Check sheet for the modelled part. Datum: model origin and axes. Units: mm. Face numbers are marked on the shaded views. A direction names the side the tool comes from. Round coordinates to 2 decimals unless told otherwise and drop trailing zeros. Order: outer loops, then holes, each group sorted by start corner. A loop starts at its lowest first (then second) coordinate and runs counter-clockwise, first axis right, second up. Notation, with made-up numbers: (-3.5, -11.5) -> (53.5, -11.5) arc R20 ccw to (53.5, 6.5) -> close; hole circle Ø9 at (89.25, 35.25). An arc over 180 degrees is marked (long way). Answer as CSV lines item,"result". Start each with the question number.
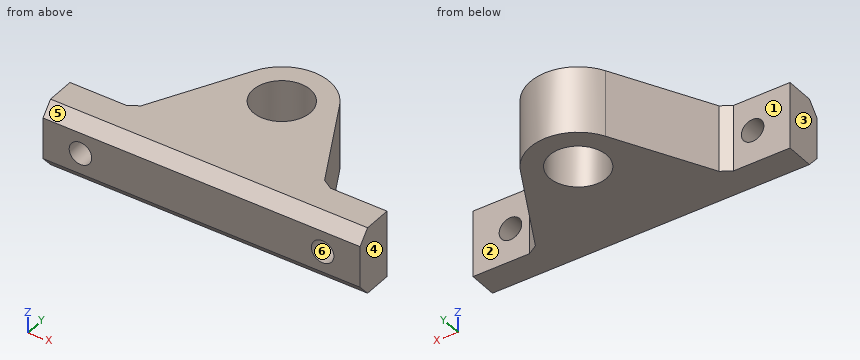
from build123d import *

# Parameters (mm, degrees)
SKETCH_R     = 4.06
PAD_DEPTH    = 9.48
PAD001_DEPTH = 45
SKETCH002_R  = 1.6
POCKET_DEPTH = 23.37485
CHAMFER_SIZE = 1


with BuildPart() as part:
    # Sketch → Pad (new body)
    with BuildSketch(Plane.XY):
        with BuildLine():
            ThreePointArc((6.02785, 14.177039), (0, 17.81385), (-6.02785, 14.177039))
            Line((-6.02785, 14.177039), (-13.5, 0))
            Line((-13.5, 0), (-22.5, 0))
            Line((-22.5, 0), (-22.5, -4))
            Line((-22.5, -4), (22.5, -4))
            Line((22.5, -4), (22.5, 0))
            Line((22.5, 0), (13.5, 0))
            Line((6.02785, 14.177039), (13.5, 0))
        make_face()
        with Locations((0, 11)):
            Circle(SKETCH_R, mode=Mode.SUBTRACT)
    extrude(amount=PAD_DEPTH)

    # Sketch001 (on Face4 of Pad) → Pad001 (join)
    with BuildSketch(Plane(origin=(-22.5, 0, 0), x_dir=(0, -1, 0), z_dir=(-1, 0, 0))):
        Polygon((4, 9.48), (4, 0), (5.56, 1.8), (5.56, 7.68), align=None)
    extrude(amount=-PAD001_DEPTH)

    # Sketch002 (on Face14 of Pad001) → Pocket (cut, through all)
    with BuildSketch(Plane.XZ.offset(5.56)):
        with Locations((-17.186, 4.74)):
            Circle(SKETCH002_R)
        with Locations((17.186, 4.74)):
            Circle(SKETCH002_R)
    extrude(amount=-POCKET_DEPTH, mode=Mode.SUBTRACT)

    # Chamfer
    chamfer_edges = [part.edges().sort_by_distance(p)[0] for p in [
        (13.5, 0, 4.74),
        (-13.5, 0, 4.74),
    ]]
    chamfer(chamfer_edges, length=CHAMFER_SIZE)


solid = part.part
1) Section check C-C on z = 7. Record the cut outline in (x, y), then the cut area to 3 significant figures.
2) Material ranges on line 1 along Y through (x, z) = (0, 2.75); line 2 along Y through (x, z) = (3, 0.5); line 3 along Y through (x, z) = (-16.5, 3), recorded low to high.
3) Section check B-B on x = 0. Record the cut outline in (y, z).
4) Section check D-D on y = -3.25. Record the cut outline in (x, z).
5) Access from +Z, -Z, +X, -X, +Y, -Y to the whole of each face (thin tool, end or side, straight path). Record for the marked faces 1, 2 and 3.
6) Section check A-A on z = 4. Record the cut outline in (x, y), then the cut area to 3 significant figures.
7) Mould release check, pull along X, two halves, no side actions. Record for the marked faces 4, 5 and 6: released by +X, released by -X, zero draft, split by the parting line, or undercut.
8) Depth check by flat-ended pin: pin 1 Ø5 at (x, z) = (-17.186, 4.74) entering from +Y; pin 2 Ø2 at (y, z) = (3.5, 1.5) entering from +X; pin 3 Ø2 at (y, z) = (12, 6.5) entering from +X. Enter the tip coordinate at first touch or a pass-through.
Solutions:
1,outline,"(-22.5, -5.56) -> (22.5, -5.56) -> (22.5, 0) -> (14.5, 0) -> (13.03, 0.88) -> (6.03, 14.18) arc R6.81 ccw to (-6.03, 14.18) -> (-13.03, 0.88) -> (-14.5, 0) -> (-22.5, 0) -> close; hole circle Ø8.12 at (0, 11)"
1,area,"507 mm^2"
2,line 1,"y = -5.56 to 6.94, 15.06 to 17.81"
2,line 2,"y = -4.43 to 8.26, 13.74 to 17.12"
2,line 3,"y = -5.56 to 0"
3,outline,"(-5.56, 1.8) -> (-4, 0) -> (6.94, 0) -> (6.94, 9.48) -> (-4, 9.48) -> (-5.56, 7.68) -> close; (15.06, 0) -> (17.81, 0) -> (17.81, 9.48) -> (15.06, 9.48) -> close"
4,outline,"(-22.5, 0) -> (22.5, 0) -> (22.5, 9.48) -> (-22.5, 9.48) -> close; hole circle Ø3.2 at (-17.19, 4.74); hole circle Ø3.2 at (17.19, 4.74)"
5,face 1,"+Z, -Z, -X, +Y"
5,face 2,"+Z, -Z, +X, +Y"
5,face 3,"+Z, -Z, -X, +Y, -Y"
6,outline,"(-22.5, -5.56) -> (-18.6, -5.56) -> (-18.6, 0) -> (-22.5, 0) -> close; (-15.77, -5.56) -> (15.77, -5.56) -> (15.77, 0) -> (14.5, 0) -> (13.03, 0.88) -> (6.03, 14.18) arc R6.81 ccw to (-6.03, 14.18) -> (-13.03, 0.88) -> (-14.5, 0) -> (-15.77, 0) -> close; (18.6, -5.56) -> (22.5, -5.56) -> (22.5, 0) -> (18.6, 0) -> close; hole circle Ø8.12 at (0, 11)"
6,area,"476 mm^2"
7,face 4,"released by +X"
7,face 5,"zero draft"
7,face 6,"undercut"
8,pin 1,"stops at y = 0"
8,pin 2,"stops at x = 12.18"
8,pin 3,"stops at x = 7.7"
